```python
from build123d import *

# Parameters (mm, degrees)
F0_W     = 42
F0_H     = 44.9056578597
F0_R     = 1.5
F0_R_2   = 11
F0_R_3   = 2.5
F1_DEPTH = 35
F2_DEPTH = 2
F3_DEPTH = 25
F4_D     = 2.4
F4_DEPTH = 19.05
F4_TIP   = 0.7210327428
F5_R     = 8


with BuildPart() as f1:
    # F0 (on Top) → F1 (new body)
    with BuildSketch(Plane.XY):
        Rectangle(F0_W, F0_H)
        with Locations((-14, -15.4528289299)):
            Circle(F0_R, mode=Mode.SUBTRACT)
        with Locations((14, -15.4528289299)):
            Circle(F0_R, mode=Mode.SUBTRACT)
        Circle(F0_R_2, mode=Mode.SUBTRACT)
        with Locations((-14, 15.4528289299)):
            Circle(F0_R, mode=Mode.SUBTRACT)
        with Locations((14, 15.4528289299)):
            Circle(F0_R, mode=Mode.SUBTRACT)
        with Locations((-14, -15.4528289299)):
            Circle(F0_R)
        Circle(F0_R_2)
        Circle(F0_R_3, mode=Mode.SUBTRACT)
        Circle(F0_R_3)
        with Locations((14, -15.4528289299)):
            Circle(F0_R)
        with Locations((-14, 15.4528289299)):
            Circle(F0_R)
        with Locations((14, 15.4528289299)):
            Circle(F0_R)
    extrude(amount=-F1_DEPTH)

    # F0 (on Top) → F2 (join)
    with BuildSketch(Plane.XY):
        Circle(F0_R_2)
        Circle(F0_R_3, mode=Mode.SUBTRACT)
        Circle(F0_R_3)
    extrude(amount=F2_DEPTH)

    # F0 (on Top) → F3 (join)
    with BuildSketch(Plane.XY):
        Circle(F0_R_3)
    extrude(amount=F3_DEPTH)

    # F4
    with Locations(Plane.XY):
        with Locations((-14, 15.4528289299), (14, 15.4528289299), (14, -15.4528289299), (-14, -15.4528289299)):
            Hole(F4_D / 2, depth=F4_DEPTH)
            with Locations((0, 0, -(F4_DEPTH + F4_TIP / 2))):  # 118° drill point
                Cone(0, F4_D / 2, F4_TIP, mode=Mode.SUBTRACT)

    # F5
    f5_edges = [f1.edges().sort_by_distance(p)[0] for p in [
        (21, 22.452829, -17.5),
        (21, -22.452829, -17.5),
        (-21, 22.452829, -17.5),
        (-21, -22.452829, -17.5),
    ]]
    fillet(f5_edges, radius=F5_R)


solid = f1.part
```
Work out the finished part from the listing and answer in its coordinate system (mm). A direction names the side the tool comes from. Coordinates: 2 decimals unless noted, no trailing zeros. Write each loop counter-clockwise with the first axis right and the second up, starting at its lowest first coordinate (ties: lowest second). Pieces come first, ordered by that corner, then holes. Notation, with made-up numbers: (42, -27) - (81, -27) arc R17 cw to (81, -12) - close; hole circle Ø5 at (78.5, -23). An arc over 180 degrees is marked (long way). Answer as a JSON object with one key per item and string values.
Q1. Find section D-D (z = -27). Write down the section's boundary in (x, y).
Results list:
{"outline": "(-21, -14.45) arc R8 ccw to (-13, -22.45) - (13, -22.45) arc R8 ccw to (21, -14.45) - (21, 14.45) arc R8 ccw to (13, 22.45) - (-13, 22.45) arc R8 ccw to (-21, 14.45) - close"}
Q2. Find section A-A (z = -2.5). Write down the section's boundary in (x, y).
Results list:
{"outline": "(-21, -14.45) arc R8 ccw to (-13, -22.45) - (13, -22.45) arc R8 ccw to (21, -14.45) - (21, 14.45) arc R8 ccw to (13, 22.45) - (-13, 22.45) arc R8 ccw to (-21, 14.45) - close; hole circle Ø2.4 at (-14, -15.45); hole circle Ø2.4 at (-14, 15.45); hole circle Ø2.4 at (14, -15.45); hole circle Ø2.4 at (14, 15.45)"}
Q3. Given pin 1 Ø17.5 at (x, y) = (2, 4.5) entering from +Z; pin 2 Ø12.5 at (x, y) = (-5, -8) entering from +Z, each flat-ended and moving along its own axis, determine where each tip first touches the part or whether it passes through.
Results list:
{"pin 1": "stops at z = 25", "pin 2": "stops at z = 2"}
Q4. Find section C-C (x = 0). Write down the section's boundary in (y, z).
Results list:
{"outline": "(-22.45, -35) - (22.45, -35) - (22.45, 0) - (11, 0) - (11, 2) - (2.5, 2) - (2.5, 25) - (-2.5, 25) - (-2.5, 2) - (-11, 2) - (-11, 0) - (-22.45, 0) - close"}
Q5. Find section B-B (y = 0). Write down the section's boundary in (x, z), plus the area to 3 significant figures.
Results list:
{"outline": "(-21, -35) - (21, -35) - (21, 0) - (11, 0) - (11, 2) - (2.5, 2) - (2.5, 25) - (-2.5, 25) - (-2.5, 2) - (-11, 2) - (-11, 0) - (-21, 0) - close", "area": "1,630 mm^2"}
Q6. Which of the six approach directions +Z, -Z, +X, -X, +Y, -Y give full straight-line access (tool end or side, diameter ignored) to faces 1 (the cylindrical face through (-0.54, -2.44, 13.34)), 2 (the flat face through (0, 0, 25))?
Results list:
{"face 1": "+Z", "face 2": "+Z, +X, -X, +Y, -Y"}
Q7. Consider L1, parallel to Y at x = 14, z = -4; L2, parallel to Z at x = -13, y = -2.5; L3, parallel to X at y = -18, z = -3. Determine where each line is inside the solid, lowest interval first. Write a range as from..to.
Results list:
{"L1": "y = -22.39..-16.65, -14.25..14.25, 16.65..22.39", "L2": "z = -35..0", "L3": "x = -20.17..20.17"}
